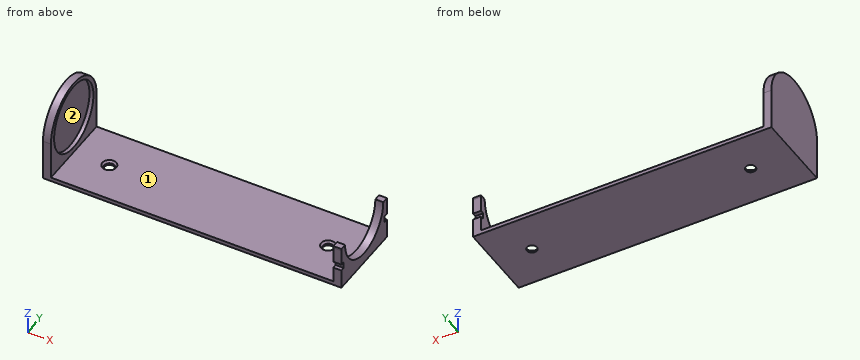
```python
from build123d import *

# Parameters (mm, degrees)
F0_W      = 150
F0_H      = 40
F1_DEPTH  = 2
F2_W      = 4
F2_H      = 40
F2_W_2    = 2
F3_DEPTH  = 40
F4_R      = 17.25
F5_DEPTH  = 2
F7_DEPTH  = 20
F8_DEPTH  = 2.001
F9_R      = 2.5
F10_DEPTH = 42.001
F11_W     = 2
F11_H     = 3.3180480823
F12_DEPTH = 25
F14_DEPTH = 150.001
F15_SIZE  = 1
F16_DEPTH = 2


with BuildPart() as f1:
    # F0 (on Top) → F1 (new body)
    with BuildSketch(Plane.XY):
        with Locations((29.9631836727, -6.3660135493)):
            Rectangle(F0_W, F0_H)
    extrude(amount=F1_DEPTH)

    # F2 (on face) → F3 (join)
    with BuildSketch(Plane.XY.offset(2)):
        with Locations((-43.0368163273, -6.3660135493)):
            Rectangle(F2_W, F2_H)
        with Locations((103.9631836727, -6.3660135493)):
            Rectangle(F2_W_2, F2_H)
    extrude(amount=F3_DEPTH)

    # F4 (on face) → F5 (cut)
    with BuildSketch(Plane.YZ.offset(-41.0368163273)):
        with Locations((-6.3660135493, 22)):
            Circle(F4_R)
    extrude(amount=-F5_DEPTH, mode=Mode.SUBTRACT)

    # F7 (cut): a face of the model
    f7_faces = [f1.faces().sort_by_distance(p)[0] for p in [
        (103.9631836727, -6.3660135493, 42),
    ]]
    extrude(f7_faces, amount=-F7_DEPTH, mode=Mode.SUBTRACT)

    # F6 (on face) → F8 (cut, through all)
    with BuildSketch(Plane(origin=(102.9631836727, 0, 0), x_dir=(0, -1, 0), z_dir=(-1, 0, 0))):
        with BuildLine():
            Line((23.1160135493, 22), (-10.3839864507, 22))
            ThreePointArc((-10.3839864507, 22), (6.3660135493, 5.25), (23.1160135493, 22))
        make_face()
    extrude(amount=-F8_DEPTH, mode=Mode.SUBTRACT)

    # F9 (on face) → F10 (cut, through all)
    with BuildSketch(Plane(origin=(0, 0, 0), x_dir=(1, 0, 0), z_dir=(0, 0, -1))):
        with Locations((-23.1661424041, 6.3660135493)):
            Circle(F9_R)
        with Locations((86.8019685149, 6.3660135493)):
            Circle(F9_R)
    extrude(amount=-F10_DEPTH, mode=Mode.SUBTRACT)

    # F11 (on face) → F12 (cut)
    with BuildSketch(Plane.YZ.offset(104.9631836727)):
        with Locations((-25.3660135493, 11.4577081986)):
            Rectangle(F11_W, F11_H)
        with Locations((12.6339864507, 11.4577081986)):
            Rectangle(F11_W, F11_H)
    extrude(amount=-F12_DEPTH, mode=Mode.SUBTRACT)

    # F13 (on face) → F14 (cut, through all)
    with BuildSketch(Plane(origin=(-45.0368163273, 0, 0), x_dir=(0, -1, 0), z_dir=(-1, 0, 0))):
        with BuildLine():
            ThreePointArc((-13.6339864507, 21), (6.3660135493, 41), (26.3660135493, 21))
            Line((26.3660135493, 21), (26.3660135493, 42))
            Line((26.3660135493, 42), (-13.6339864507, 42))
            Line((-13.6339864507, 42), (-13.6339864507, 21))
        make_face()
    extrude(amount=-F14_DEPTH, mode=Mode.SUBTRACT)

    # F15
    f15_edges = [f1.edges().sort_by_distance(p)[0] for p in [
        (-25.666142, -6.366014, 2),
        (84.301969, -6.366014, 2),
    ]]
    chamfer(f15_edges, length=F15_SIZE)

    # F16 (add): a face of the model
    f16_faces = [f1.faces().sort_by_distance(p)[0] for p in [
        (102.9631836727, -6.3660135493, 2.4472135955),
    ]]
    extrude(f16_faces, amount=F16_DEPTH)


solid = f1.part
```
Could you check a few things on this model? Use its own coordinates, in mm. Face numbers are marked on the shaded views. Give positions to 0.01 mm unless a question says otherwise; leave off trailing zeros. Order: outer loops, then holes, each group sorted by start corner. A loop starts at its lowest first (then second) coordinate and runs counter-clockwise, first axis right, second up.
Q1. If I drill on line 1 along X through (y, z) = (-23, 18.5); line 2 along X through (y, z) = (3, 28.5); line 3 along X through (y, z) = (-23, 9.5), over which ranges is the centre line in solid material (lowest first)?
Q2. Suppose I cut it at C-C, the plane y = -12. Write out the boundary of the cut face in (x, z), and give its area (3 significant figures).
Q3. Suppose I cut it at B-B, the plane x = 29.5. Write out the boundary of the cut face in (y, z).
Q4. We'd pull the mould along Y, two halves only. Please class the marked faces 1 and 2: +Y half, -Y half, draft (parallel to the pull), parting line (faces both ways), or undercut.
Q5. Suppose I cut it at D-D, the plane z = 36. Write out the boundary of the cut face in (x, y), and give its area (3 significant figures).
Q6. Suppose I cut it at A-A, the plane z = 27.5. Write out the boundary of the cut face in (x, y), and give its area (3 significant figures).
Q7. I'm going to push flat-ended pins straight in: P1, Ø1, axis at x = 49, y = 3.5, coming from the +Z side; P2, Ø2, axis at x = 102.5, y = 13, coming from the -Z side; P3, Ø6, axis at x = -23.17, y = -6.37, coming from the +Z side; P4, Ø1, axis at x = 102.5, y = -25, coming from the +Z side. Where does each tip first touch, or does it pass through?
Solution:
1. line 1: x = -45.04 to -43.04, 100.96 to 104.96
1. line 2: x = -45.04 to -43.04
1. line 3: x = -45.04 to -41.04, 100.96 to 104.96
2. outline: (-45.04, 0) - (104.96, 0) - (104.96, 6.23) - (100.96, 6.23) - (100.96, 2) - (-41.04, 2) - (-41.04, 5.7) - (-43.04, 5.7) - (-43.04, 38.3) - (-41.04, 38.3) - (-41.04, 40.19) - (-45.04, 40.19) - close
2. area: 404 mm2
3. outline: (-26.37, 0) - (13.63, 0) - (13.63, 2) - (-26.37, 2) - close
4. face 1: draft
4. face 2: undercut
5. outline: (-45.04, -19.59) - (-41.04, -19.59) - (-41.04, -16.44) - (-43.04, -16.44) - (-43.04, 3.71) - (-41.04, 3.71) - (-41.04, 6.86) - (-45.04, 6.86) - close
5. area: 65.5 mm2
6. outline: (-45.04, -25.28) - (-41.04, -25.28) - (-41.04, -22.72) - (-43.04, -22.72) - (-43.04, 9.98) - (-41.04, 9.98) - (-41.04, 12.55) - (-45.04, 12.55) - close
6. area: 85.9 mm2
7. P1: stops at z = 2
7. P2: stops at z = 0
7. P3: stops at z = 1.51
7. P4: stops at z = 22
